Read the model definition and answer for the solid it produces. Units are mm, in the model's axes. Face numbers are marked on the shaded views. Coordinates: 2 decimals unless noted, no trailing zeros. Use a Markdown table: item, result.
from build123d import *

# Parameters (mm, degrees)
CYLINDER037_R               = 1.25
CYLINDER037_DEPTH           = 14
CYLINDER037_ROLL_ANGLE      = -89.999776
CYLINDER037_PITCH_ANGLE     = 1.4e-05
CYLINDER037_PLACEMENT_ANGLE = -9.999925
CYLINDER029_R               = 3
CYLINDER029_DEPTH           = 14
CYLINDER029_ROLL_ANGLE      = -89.999776
CYLINDER029_PITCH_ANGLE     = 1.4e-05
CYLINDER029_PLACEMENT_ANGLE = -9.999925


with BuildPart() as cylinder037:
    # Cylinder037 → Cylinder037 (new body)
    with BuildSketch(Plane.XY):
        Circle(CYLINDER037_R)
    extrude(amount=CYLINDER037_DEPTH)


with BuildPart() as cylinder037_1:
    # Cylinder037 roll: moved
    add(cylinder037.part.rotate(Axis((0, 0, 0), (1, 0, 0)), CYLINDER037_ROLL_ANGLE))


with BuildPart() as cylinder037_2:
    # Cylinder037 pitch: moved
    add(cylinder037_1.part.rotate(Axis((0, 0, 0), (0, 1, 0)), CYLINDER037_PITCH_ANGLE))


with BuildPart() as cylinder037_3:
    # Cylinder037 placement: moved
    add(cylinder037_2.part.moved(Location((39.936521, -25.15501, 25.500007))).rotate(Axis((39.936521, -25.15501, 25.500007), (0, 0, 1)), CYLINDER037_PLACEMENT_ANGLE))


with BuildPart() as cut034:
    # Cylinder029 → Cylinder029 (new body)
    with BuildSketch(Plane.XY):
        Circle(CYLINDER029_R)
    extrude(amount=CYLINDER029_DEPTH)


with BuildPart() as cut034_1:
    # Cylinder029 roll: moved
    add(cut034.part.rotate(Axis((0, 0, 0), (1, 0, 0)), CYLINDER029_ROLL_ANGLE))


with BuildPart() as cut034_2:
    # Cylinder029 pitch: moved
    add(cut034_1.part.rotate(Axis((0, 0, 0), (0, 1, 0)), CYLINDER029_PITCH_ANGLE))


with BuildPart() as cut034_3:
    # Cylinder029 placement: moved
    add(cut034_2.part.moved(Location((39.589228, -27.124626, 25.499999))).rotate(Axis((39.589228, -27.124626, 25.499999), (0, 0, 1)), CYLINDER029_PLACEMENT_ANGLE))

    # Cut034: cut Cylinder037
    add(cylinder037_3.part, mode=Mode.SUBTRACT)


solid = cut034_3.part
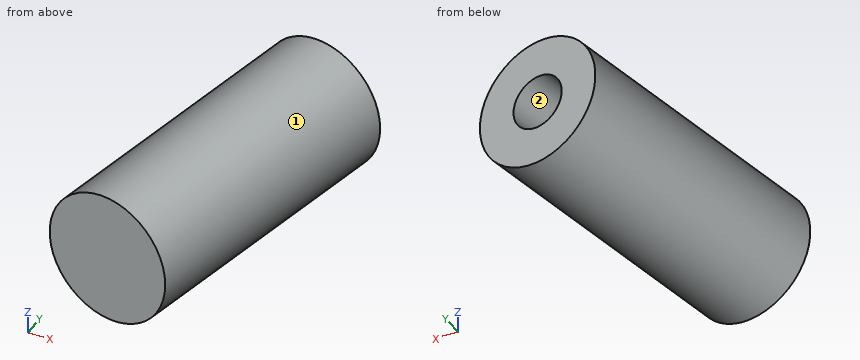
(1) The mould has two halves that part along Y. Classify the marked faces 1 and 2: pulls with the +Y half, pulls with the -Y half, needs draft (parallel to the pull), parting line crosses it, or undercut.
Report:
| item | result |
|---|---|
| face 1 | parting line crosses it |
| face 2 | undercut |
(2) Each of these flat-tipped pins is pushed along its axis until it touches: P1, Ø1, axis at x = 41, z = 24.5, coming from the -Y side; P2, Ø4, axis at x = 37.5, y = -23, coming from the +Z side. Where does it stop, or does it pass through?
Report:
| item | result |
|---|---|
| P1 | stops at y = -27.46 |
| P2 | stops at z = 28.4 |
(3) Straight lines are drawn through the part: L1, parallel to Z at x = 40.5, y = -21.5; L2, parallel to X at y = -17.25, z = 26.25; L3, parallel to X at y = -23.5, z = 25.25. For each, find the intervals that lie inside material, in ascending order.
Report:
| item | result |
|---|---|
| L1 | z = 22.5 to 24.25, 26.75 to 28.5 |
| L2 | x = 38.38 to 40.31, 42.35 to 44.28 |
| L3 | x = 37.19 to 38.98, 41.47 to 43.26 |
